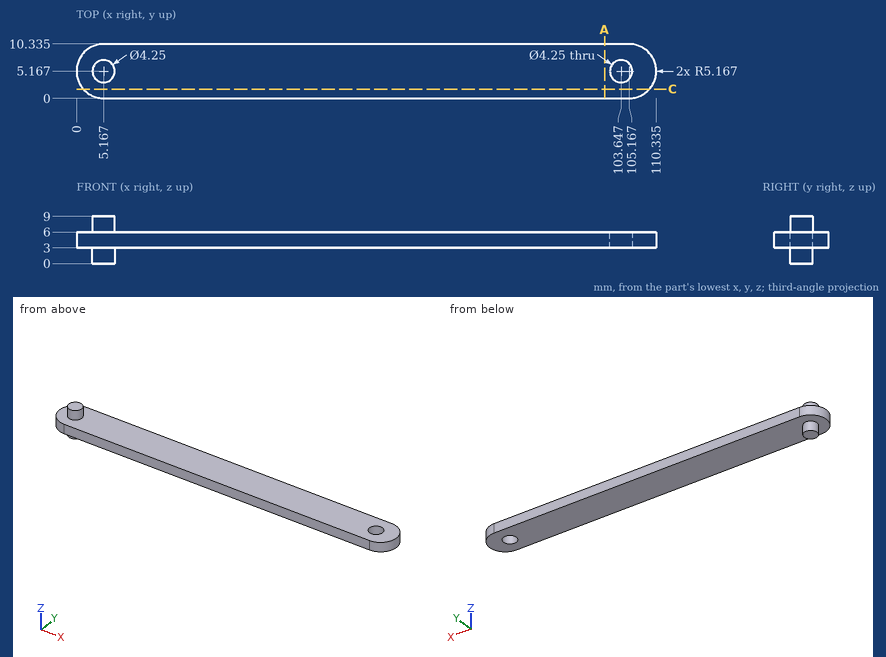
Here's the drawing with two shaded views (mm, measured from the low corner). I have some questions. Coordinates: 2 decimals unless noted, no trailing zeros. Write each loop counter-clockwise with the first axis right and the second up, starting at its lowest first coordinate (ties: lowest second). Pieces come first, ordered by that corner, then holes. Notation, with made-up numbers: M -26,72 L 20,72 A22 ccw 20,99 Z; hole C 41.5,-24 d8. An arc over 180 degrees is marked long. Use one line per item in the form item = value.
Q1. If we section it at C-C (y = 1.75): Write out the boundary of the cut face in (x, z).
Model answer:
outline = M 1.29,3 L 109.04,3 L 109.04,6 L 1.29,6 Z
Q2. For P1, Ø5, axis at x = 48.5, y = 5, coming from the -Z side; P2, Ø2, axis at x = 46.5, y = 6, coming from the +Z side, each with a flat end and sliding along its axis, tell me the tip position at first contact or that it passes through.
Model answer:
P1 = 3
P2 = 6
Q3. If we section it at A-A (x = 100.5): Write out the boundary of the cut face in (y, z) (1 decimal), then the cut area to 3 significant figures.
Model answer:
outline = M 0,3 L 10.3,3 L 10.3,6 L 0,6 Z
area = 31.0 mm^2
Q4. I need wall thicknesses on line 1 along Z through (x, y) = (32.5, 6.75); line 2 along X through (y, z) = (5, 1) (1 decimal); line 3 along X through (y, z) = (6.5, 4) (1 decimal). Which ranges of each line are inside material? Lowest first, please. Write a range as from..to.
Model answer:
line_1 = 3..6
line_2 = 3..7.3
line_3 = 0.2..102, 105.3..110.2
